from build123d import *

# Parameters (mm, degrees)
SKETCH_1_W      = 2
SKETCH_1_H      = 40
SKETCH_1_W_2    = 40
SKETCH_1_H_2    = 2
SKETCH_1_W_3    = 50
SKETCH_1_R      = 15
SKETCH_1_W_4    = 30
EXTRUDE_3_DEPTH = 2
EXTRUDE_4_DEPTH = 12


with BuildPart() as part:
    # 草图1 → 凸台-拉伸3 (new body)
    with BuildSketch(Plane(origin=(0, 0, 0), x_dir=(0, 0, -1), z_dir=(1, 0, 0))):
        with BuildLine():
            ThreePointArc((0, 51), (-51, 0), (0, -51))
            Line((0, -51), (350, -51))
            Line((350, -51), (350, -20))
            Line((350, -20), (352, -20))
            Line((352, -20), (352, 20))
            Line((352, 20), (350, 20))
            Line((350, 20), (350, 51))
            Line((350, 51), (0, 51))
        make_face()
        with Locations((1, 0)):
            Rectangle(SKETCH_1_W, SKETCH_1_H, mode=Mode.SUBTRACT)
        with Locations((60, -41)):
            Rectangle(SKETCH_1_W_2, SKETCH_1_H_2, mode=Mode.SUBTRACT)
        with BuildLine():
            Line((35.191745563, -17.73919947), (35.191745563, 7.047932671))
            ThreePointArc((35.191745563, 7.047932671), (35.944654473, 8.3486459), (37.447552101, 8.343601023))
            Line((37.447552101, 8.343601023), (58.776761956, -4.098438059))
            ThreePointArc((58.776761956, -4.098438059), (59.520953252, -5.396654882), (58.772354967, -6.69233548))
            Line((58.772354967, -6.69233548), (37.443145112, -19.03742854))
            ThreePointArc((37.443145112, -19.03742854), (35.942445664, -19.038641528), (35.191745563, -17.73919947))
        make_face(mode=Mode.SUBTRACT)
        with BuildLine():
            Line((89.643364708, -25.34051183), (45.740126418, -25.34051183))
            ThreePointArc((45.740126418, -25.34051183), (44.292110098, -24.231981799), (44.98431988, -22.544843479))
            Line((44.98431988, -22.544843479), (66.935939025, -9.739732311))
            ThreePointArc((66.935939025, -9.739732311), (67.691745563, -9.535400662), (68.447552101, -9.739732311))
            Line((68.447552101, -9.739732311), (90.399171246, -22.544843479))
            ThreePointArc((90.399171246, -22.544843479), (91.091381028, -24.231981799), (89.643364708, -25.34051183))
        make_face(mode=Mode.SUBTRACT)
        with BuildLine():
            ThreePointArc((97.935939025, 8.343601023), (99.438836653, 8.3486459), (100.191745563, 7.047932671))
            Line((100.191745563, 7.047932671), (100.191745563, -17.728956331))
            ThreePointArc((100.191745563, -17.728956331), (99.438836653, -19.02966956), (97.935939025, -19.024624683))
            Line((97.935939025, -19.024624683), (76.698605594, -6.636180181))
            ThreePointArc((76.698605594, -6.636180181), (75.954412132, -5.34051183), (76.698605594, -4.044843479))
            Line((76.698605594, -4.044843479), (97.935939025, 8.343601023))
        make_face(mode=Mode.SUBTRACT)
        with BuildLine():
            Line((135, -17.73919947), (135, 7.047932671))
            ThreePointArc((135, 7.047932671), (135.75290891, 8.3486459), (137.255806538, 8.343601023))
            Line((137.255806538, 8.343601023), (158.585016393, -4.098438059))
            ThreePointArc((158.585016393, -4.098438059), (159.329207689, -5.396654882), (158.580609404, -6.69233548))
            Line((158.580609404, -6.69233548), (137.25139955, -19.03742854))
            ThreePointArc((137.25139955, -19.03742854), (135.750700102, -19.038641528), (135, -17.73919947))
        make_face(mode=Mode.SUBTRACT)
        with Locations((175, -41)):
            Rectangle(SKETCH_1_W_3, SKETCH_1_H_2, mode=Mode.SUBTRACT)
        with Locations((295, -41)):
            Rectangle(SKETCH_1_W_3, SKETCH_1_H_2, mode=Mode.SUBTRACT)
        with BuildLine():
            Line((189.451619145, -25.34051183), (145.548380855, -25.34051183))
            ThreePointArc((145.548380855, -25.34051183), (144.100364535, -24.231981799), (144.792574317, -22.544843479))
            Line((144.792574317, -22.544843479), (166.744193462, -9.739732311))
            ThreePointArc((166.744193462, -9.739732311), (167.5, -9.535400662), (168.255806538, -9.739732311))
            Line((168.255806538, -9.739732311), (190.207425683, -22.544843479))
            ThreePointArc((190.207425683, -22.544843479), (190.899635465, -24.231981799), (189.451619145, -25.34051183))
        make_face(mode=Mode.SUBTRACT)
        with BuildLine():
            ThreePointArc((197.744193462, 8.684112853), (199.24709109, 8.68915773), (200, 7.388444501))
            Line((200, 7.388444501), (200, -17.388444501))
            ThreePointArc((200, -17.388444501), (199.24709109, -18.68915773), (197.744193462, -18.684112853))
            Line((197.744193462, -18.684112853), (176.506860031, -6.295668351))
            ThreePointArc((176.506860031, -6.295668351), (175.762666569, -5), (176.506860031, -3.704331649))
            Line((176.506860031, -3.704331649), (197.744193462, 8.684112853))
        make_face(mode=Mode.SUBTRACT)
        with Locations((232.5, -5)):
            Circle(SKETCH_1_R, mode=Mode.SUBTRACT)
        with BuildLine():
            Line((319.974166797, -25.394327939), (276.070928507, -25.394327939))
            ThreePointArc((276.070928507, -25.394327939), (274.622912187, -24.285797907), (275.315121969, -22.598659587))
            Line((275.315121969, -22.598659587), (297.266741114, -9.793548419))
            ThreePointArc((297.266741114, -9.793548419), (298.022547652, -9.589216771), (298.778354191, -9.793548419))
            Line((298.778354191, -9.793548419), (320.729973336, -22.598659587))
            ThreePointArc((320.729973336, -22.598659587), (321.422183118, -24.285797907), (319.974166797, -25.394327939))
        make_face(mode=Mode.SUBTRACT)
        with BuildLine():
            Line((265.522547652, -17.793015579), (265.522547652, 6.994116563))
            ThreePointArc((265.522547652, 6.994116563), (266.275456563, 8.294829792), (267.778354191, 8.289784914))
            Line((267.778354191, 8.289784914), (289.107564045, -4.152254168))
            ThreePointArc((289.107564045, -4.152254168), (289.851755342, -5.45047099), (289.103157056, -6.746151588))
            Line((289.103157056, -6.746151588), (267.773947202, -19.091244648))
            ThreePointArc((267.773947202, -19.091244648), (266.273247754, -19.092457637), (265.522547652, -17.793015579))
        make_face(mode=Mode.SUBTRACT)
        with BuildLine():
            ThreePointArc((327.730104505, 8.28146303), (329.239985391, 8.298885363), (330, 6.994116563))
            Line((330, 6.994116563), (330, -17.477952976))
            ThreePointArc((330, -17.477952976), (329.24709109, -18.778666205), (327.744193462, -18.773621327))
            Line((327.744193462, -18.773621327), (307.029407683, -6.68999629))
            ThreePointArc((307.029407683, -6.68999629), (306.285236534, -5.40250951), (307.015318726, -4.106981472))
            Line((307.015318726, -4.106981472), (327.730104505, 8.28146303))
        make_face(mode=Mode.SUBTRACT)
        with BuildLine():
            ThreePointArc((44.98431988, 11.863819819), (44.292110098, 13.550958139), (45.740126418, 14.65948817))
            Line((45.740126418, 14.65948817), (90.076891362, 14.65948817))
            ThreePointArc((90.076891362, 14.65948817), (91.525570692, 13.548497422), (90.828290911, 11.861259101))
            Line((90.828290911, 11.861259101), (68.573204722, -1.019720173))
            ThreePointArc((68.573204722, -1.019720173), (67.819256701, -1.221488939), (67.065998635, -1.017159455))
            Line((67.065998635, -1.017159455), (44.98431988, 11.863819819))
        make_face(mode=Mode.SUBTRACT)
        with BuildLine():
            ThreePointArc((144.792574317, 11.863819819), (144.100364535, 13.550958139), (145.548380855, 14.65948817))
            Line((145.548380855, 14.65948817), (189.885145799, 14.65948817))
            ThreePointArc((189.885145799, 14.65948817), (191.333825129, 13.548497422), (190.636545348, 11.861259101))
            Line((190.636545348, 11.861259101), (168.381459159, -1.019720173))
            ThreePointArc((168.381459159, -1.019720173), (167.627511138, -1.221488939), (166.874253072, -1.017159455))
            Line((166.874253072, -1.017159455), (144.792574317, 11.863819819))
        make_face(mode=Mode.SUBTRACT)
        with BuildLine():
            ThreePointArc((275.298059327, 12.21443661), (274.625531488, 13.901032988), (276.070928507, 15))
            Line((276.070928507, 15), (321.088992758, 15))
            ThreePointArc((321.088992758, 15), (322.537672089, 13.889009252), (321.840392308, 12.20177093))
            Line((321.840392308, 12.20177093), (298.904006812, -1.073536282))
            ThreePointArc((298.904006812, -1.073536282), (298.140143671, -1.275255431), (297.379738082, -1.060870603))
            Line((297.379738082, -1.060870603), (275.298059327, 12.21443661))
        make_face(mode=Mode.SUBTRACT)
        with BuildLine():
            Line((95, 37), (95, 39))
            ThreePointArc((95, 39), (96.757359313, 43.242640687), (101, 45))
            Line((101, 45), (185, 45))
            Line((185, 45), (185, 45.8))
            Line((185, 45.8), (255, 45.8))
            Line((255, 45.8), (255, 45))
            Line((255, 45), (275.5, 45))
            ThreePointArc((275.5, 45), (279.742640687, 43.242640687), (281.5, 39))
            Line((281.5, 39), (281.5, 31))
            Line((281.5, 31), (101, 31))
            ThreePointArc((101, 31), (96.757359313, 32.757359313), (95, 37))
        make_face(mode=Mode.SUBTRACT)
        Polygon((-40, 20), (-9.698170842, 42.091834457), (-8.519939671, 40.475736902), (-38.821768829, 18.383902445), align=None, mode=Mode.SUBTRACT)
        with Locations((-25, -9)):
            Rectangle(SKETCH_1_W_4, SKETCH_1_H_2, mode=Mode.SUBTRACT)
        Polygon((-40, -20), (-38.821768829, -18.383902445), (-8.519939671, -40.475736902), (-9.698170842, -42.091834457), align=None, mode=Mode.SUBTRACT)
    extrude(amount=EXTRUDE_3_DEPTH)

    # 草图2 → 凸台-拉伸4 (add)
    with BuildSketch(Plane(origin=(0, 0, 0), x_dir=(0, 0, -1), z_dir=(1, 0, 0))):
        Polygon((101, 51), (101, 45), (185, 45), (185, 45.8), (255, 45.8), (255, 45), (276, 45), (276, 51), align=None)
    extrude(amount=EXTRUDE_4_DEPTH)


solid = part.part
The model under review builds one solid part; all positions refer to its coordinate system, in mm. Coordinates: 2 decimals unless noted, no trailing zeros. Loops run counter-clockwise (first coordinate to the right, second up) from the corner with the lowest first, then second, coordinate; pieces in that order, holes last. Notation, with made-up numbers: (61.5, 51.5) -> (93.5, 51.5) arc R17 ccw to (93.5, 77.5) -> close; hole circle Ø2 at (-38.75, 78). An arc over 180 degrees is marked (long way). Use a Markdown table: item, result. Add a question column.
1. To check wall thickness, follow line 1 (Y direction, x = 0.6, z = -232.5); line 2 (X direction, y = 28.5, z = 15); line 3 (Y direction, x = 1.5, z = 35). State the ranges of each line that lie inside material, in increasing order.
2. Draft analysis for pull direction Y (two halves, no side actions). For faces 1 (the face through (0.986, -12.577, -187.274)), 2 (the face through (5, 51, -177)), 3 (the face through (0.99, 30.89, 25.06)), state which applies: pulls with the +Y half, pulls with the -Y half, needs draft (parallel to the pull), parting line crosses it, or undercut.
3. Add section C-C on x = 6. Write out the cut boundary in (y, z), plus the area to 3 significant figures.
4. Add section A-A on z = -232.5. Write out the cut boundary in (x, y).
5. Add section B-B on y = -36.5. Write out the cut boundary in (x, z).
6. Clearance check with flat-ended pins moving along their axes: pin 1 Ø24 at (y, z) = (-5, -232.5) entering from +X; pin 2 Ø2 at (x, y) = (1, -1) entering from +Z; pin 3 Ø0.6 at (x, y) = (1.5, -11.5) entering from +Z (3 decimals); pin 4 Ø10 at (y, z) = (23, -304.5) entering from +X. State where each tip first meets the part, or that it passes through.
Returned:
| question | item | result |
|---|---|---|
| 1 | line 1 | y = -51 to -20, 10 to 31, 45.8 to 51 |
| 1 | line 2 | x = 0 to 2 |
| 1 | line 3 | y = -37.09 to -23.65, -21.17 to -10, -8 to 21.17, 23.65 to 37.09 |
| 2 | face 1 | undercut |
| 2 | face 2 | pulls with the +Y half |
| 2 | face 3 | undercut |
| 3 | outline | (45, -276) -> (51, -276) -> (51, -101) -> (45, -101) -> (45, -185) -> (45.8, -185) -> (45.8, -255) -> (45, -255) -> close |
| 3 | area | 994 mm² |
| 4 | outline | (0, -51) -> (2, -51) -> (2, -20) -> (0, -20) -> close; (0, 10) -> (2, 10) -> (2, 31) -> (0, 31) -> close; (0, 45.8) -> (12, 45.8) -> (12, 51) -> (0, 51) -> close |
| 5 | outline | (0, -350) -> (2, -350) -> (2, 13.97) -> (0, 13.97) -> close; (0, 17.37) -> (2, 17.37) -> (2, 35.62) -> (0, 35.62) -> close |
| 6 | pin 1 | passes through |
| 6 | pin 2 | stops at z = 51 |
| 6 | pin 3 | stops at z = 49.755 |
| 6 | pin 4 | stops at x = 2 |
